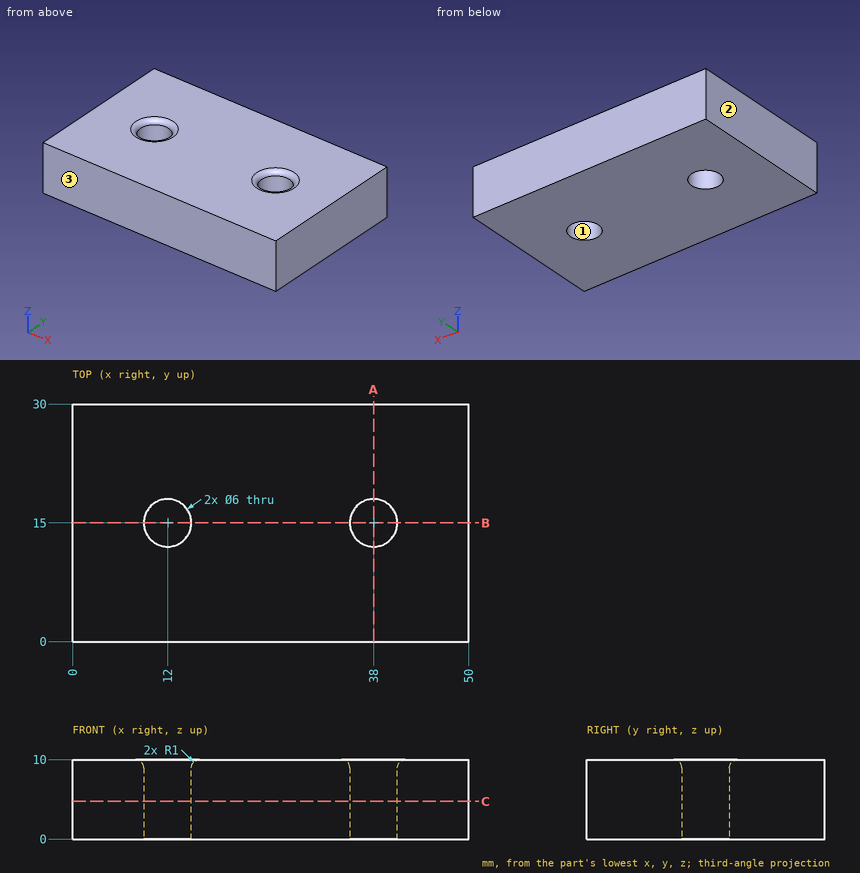
Could you check a few things on this drawing? It's one solid part, dimensions in mm from its lowest x, y, z. Coordinates: 2 decimals unless noted, no trailing zeros. Order: outer loops, then holes, each group sorted by start corner. A loop starts at its lowest first (then second) coordinate and runs counter-clockwise, first axis right, second up. Notation, with made-up numbers: M 20,-1 L 72,-1 A24 cw 72,30 Z; hole C 44.5,14 d3. An arc over 180 degrees is marked long. Use a Markdown table: item, result. Add a question column.
Q1. We'd pull the mould along X, two halves only. Please class the marked faces 1, 2 and 3: pulls with the +X half, pulls with the -X half, needs draft (parallel to the pull), parting line crosses it, or undercut.
Q2. I want a section at A-A on x = 38. List the corners of the cut face in (y, z) for me, then the cut area to 3 significant figures.
Q3. I want a section at C-C on z = 4.75. List the corners of the cut face in (x, y) for me, then the cut area to 3 significant figures.
Q4. I want a section at B-B on y = 15. List the corners of the cut face in (x, z) for me, then the cut area to 3 significant figures.
Q5. I'm going to push a flat-ended pin straight in: pin 1 (7 mm diameter, centred on x = 12, y = 15, fed in from +Z). Where does the tip first touch, or does it pass through?
Q6. If I drill on L1, parallel to X at y = 15.25, z = 2.25; L2, parallel to Y at x = 38, z = 4.25; L3, parallel to X at y = 13.25, z = 8.25, over which ranges is the centre line in solid material (lowest first)?
Checked values:
| question | item | result |
|---|---|---|
| 1 | face 1 | undercut |
| 1 | face 2 | pulls with the -X half |
| 1 | face 3 | needs draft |
| 2 | outline | M 0,0 L 12,0 L 12,9 A1 ccw 11,10 L 0,10 Z; M 18,0 L 30,0 L 30,10 L 19,10 A1 ccw 18,9 Z |
| 2 | area | 240 mm² |
| 3 | outline | M 0,0 L 50,0 L 50,30 L 0,30 Z; hole C 12,15 d6; hole C 38,15 d6 |
| 3 | area | 1,440 mm² |
| 4 | outline | M 0,0 L 9,0 L 9,9 A1 ccw 8,10 L 0,10 Z; M 15,0 L 35,0 L 35,9 A1 ccw 34,10 L 16,10 A1 ccw 15,9 Z; M 41,0 L 50,0 L 50,10 L 42,10 A1 ccw 41,9 Z |
| 4 | area | 379 mm² |
| 5 | pin 1 | z = 9.87 |
| 6 | L1 | 0 to 9.01, 14.99 to 35.01, 40.99 to 50 |
| 6 | L2 | 0 to 12, 18 to 30 |
| 6 | L3 | 0 to 9.56, 14.44 to 35.56, 40.44 to 50 |
